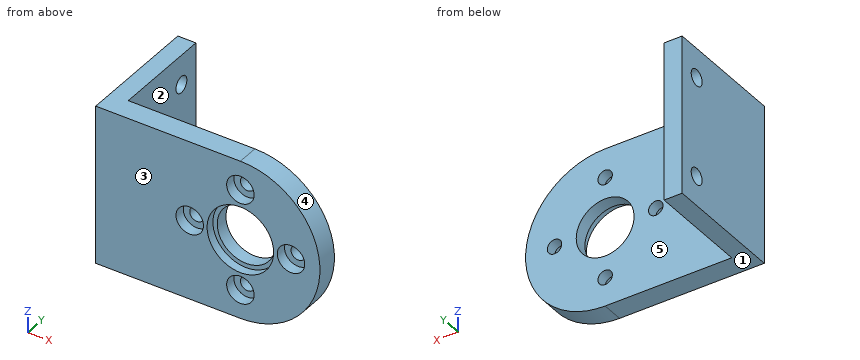
```python
from build123d import *

# Parameters (mm, degrees)
SKETCH1_R           = 1
SKETCH1_R_2         = 4
BOSS_EXTRUDE1_DEPTH = 3
SKETCH2_W           = 2.5
SKETCH2_H           = 22
BOSS_EXTRUDE2_DEPTH = 14
SKETCH3_R           = 1.132393425
SKETCH3_R_2         = 1.130977438
CUT_EXTRUDE1_DEPTH  = 6
SKETCH4_R           = 4.6
CUT_EXTRUDE2_DEPTH  = 1.2
SKETCH5_R           = 1.9
CUT_EXTRUDE3_DEPTH  = 1.5


with BuildPart() as part:
    # Sketch1 → Boss-Extrude1 (new body)
    with BuildSketch(Plane(origin=(0, 0, 0), x_dir=(1, 0, 0), z_dir=(0, 1, 0))):
        with BuildLine():
            Line((-14, -11), (-14, 11))
            Line((-14, 11), (6, 11))
            ThreePointArc((6, 11), (17, 0), (6, -11))
            Line((6, -11), (-14, -11))
        make_face()
        with Locations((6, -7)):
            Circle(SKETCH1_R, mode=Mode.SUBTRACT)
        with Locations((-1, 0)):
            Circle(SKETCH1_R, mode=Mode.SUBTRACT)
        with Locations((6, 0)):
            Circle(SKETCH1_R_2, mode=Mode.SUBTRACT)
        with Locations((13, 0)):
            Circle(SKETCH1_R, mode=Mode.SUBTRACT)
        with Locations((6, 7)):
            Circle(SKETCH1_R, mode=Mode.SUBTRACT)
    extrude(amount=BOSS_EXTRUDE1_DEPTH)

    # Sketch2 → Boss-Extrude2 (add)
    with BuildSketch(Plane(origin=(0, 3, 0), x_dir=(1, 0, 0), z_dir=(0, 1, 0))):
        with Locations((-12.75, 0)):
            Rectangle(SKETCH2_W, SKETCH2_H)
    extrude(amount=BOSS_EXTRUDE2_DEPTH)

    # Sketch3 → Cut-Extrude1 (cut)
    with BuildSketch(Plane(origin=(-11.5, 0, 0), x_dir=(0, 0, -1), z_dir=(1, 0, 0))):
        with Locations((6.9, 14)):
            Circle(SKETCH3_R)
        with Locations((-6.9, 14)):
            Circle(SKETCH3_R_2)
    extrude(amount=-CUT_EXTRUDE1_DEPTH, mode=Mode.SUBTRACT)

    # Sketch4 → Cut-Extrude2 (cut)
    with BuildSketch(Plane.XZ):
        with Locations((6, 0)):
            Circle(SKETCH4_R)
    extrude(amount=-CUT_EXTRUDE2_DEPTH, mode=Mode.SUBTRACT)

    # Sketch5 → Cut-Extrude3 (cut)
    with BuildSketch(Plane.XZ):
        with Locations((13, 0)):
            Circle(SKETCH5_R)
        with Locations((6, -7)):
            Circle(SKETCH5_R)
        with Locations((-1, 0)):
            Circle(SKETCH5_R)
        with Locations((6, 7)):
            Circle(SKETCH5_R)
    extrude(amount=-CUT_EXTRUDE3_DEPTH, mode=Mode.SUBTRACT)


solid = part.part
```
Source: CAD feature listing. Evaluate the final solid. Frame: model axes, mm. Face numbers are marked on the shaded views. A direction names the side the tool comes from. Coordinates: 2 decimals unless noted, no trailing zeros. Order: outer loops, then holes, each group sorted by start corner. A loop starts at its lowest first (then second) coordinate and runs counter-clockwise, first axis right, second up. Notation, with made-up numbers: (73, 40.5) - (132, 40.5) arc R6 cw to (132, 46.5) - close; hole circle Ø9 at (86, 14.5). An arc over 180 degrees is marked (long way). One line per item, written item: value.
1) Cut plane D-D on z = -2.25. Output: boundary loops of the cut face in (x, y), plus the area to 3 significant figures.
Computed values:
outline: (-14, 0) - (1.99, 0) - (1.99, 1.2) - (2.69, 1.2) - (2.69, 3) - (-11.5, 3) - (-11.5, 17) - (-14, 17) - close; (9.31, 1.2) - (10.01, 1.2) - (10.01, 0) - (16.77, 0) - (16.77, 3) - (9.31, 3) - close
area: 106 mm^2
2) Reachability of the marked faces 1 and 2 from +Z, -Z, +X, -X, +Y, -Y: full face, straight path, thin tool, end or side. Return the list, or none.
Computed values:
face 1: -Z, +X, -X, +Y, -Y
face 2: +Z, -Z, +X, +Y
3) Mould query, pull axis Y, two halves, no side actions, for the marked faces 3, 4 and 5. Classes: released by +Y, released by -Y, zero draft, split by the parting line, or undercut.
Computed values:
face 3: released by -Y
face 4: zero draft
face 5: released by +Y
4) Ray query, line 1 (Z direction, x = 6, y = 1.65); line 2 (X direction, y = 2.15, z = 0); line 3 (Y direction, x = -12.7, z = -6.9). Return the intervals inside material, ascending. Write a range as [from, to].
Computed values:
line 1: z = [-11, -8], [-6, -4], [4, 6], [8, 11]
line 2: x = [-14, -2], [0, 2], [10, 12], [14, 17]
line 3: y = [0, 12.87], [15.13, 17]
5) Cut plane C-C on x = 5.5. Output: boundary loops of the cut face in (y, z), plus the area to 3 significant figures.
Computed values:
outline: (0, -11) - (3, -11) - (3, -7.87) - (1.5, -7.87) - (1.5, -8.83) - (0, -8.83) - close; (0, -5.17) - (1.5, -5.17) - (1.5, -6.13) - (3, -6.13) - (3, -3.97) - (1.2, -3.97) - (1.2, -4.57) - (0, -4.57) - close; (0, 4.57) - (1.2, 4.57) - (1.2, 3.97) - (3, 3.97) - (3, 6.13) - (1.5, 6.13) - (1.5, 5.17) - (0, 5.17) - close; (0, 8.83) - (1.5, 8.83) - (1.5, 7.87) - (3, 7.87) - (3, 11) - (0, 11) - close
area: 24.5 mm^2
6) Contact query for flat-ended pins moving along their axis: pin 1 (3 mm diameter, centred on x = 13, z = 0, fed in from +Y); pin 2 (7 mm diameter, centred on x = 6, z = 0, fed in from -Y); pin 3 (3 mm diameter, centred on x = -1, z = 0, fed in from -Y); pin 4 (3 mm diameter, centred on y = 12.5, z = -2, fed in from +X). Output: stop coordinate, or through.
Computed values:
pin 1: stops at y = 3
pin 2: passes through
pin 3: stops at y = 1.5
pin 4: stops at x = -11.5
7) Cut plane B-B on y = 14. Output: boundary loops of the cut face in (x, z).
Computed values:
outline: (-14, -11) - (-11.5, -11) - (-11.5, -8.03) - (-14, -8.03) - close; (-14, -5.77) - (-11.5, -5.77) - (-11.5, 5.77) - (-14, 5.77) - close; (-14, 8.03) - (-11.5, 8.03) - (-11.5, 11) - (-14, 11) - close
8) Cut plane A-A on z = 7. Output: boundary loops of the cut face in (x, y), plus the area to 3 significant figures.
Computed values:
outline: (-14, 0) - (4.1, 0) - (4.1, 1.5) - (5, 1.5) - (5, 3) - (-11.5, 3) - (-11.5, 12.87) - (-14, 12.87) - close; (-14, 15.13) - (-11.5, 15.13) - (-11.5, 17) - (-14, 17) - close; (7, 1.5) - (7.9, 1.5) - (7.9, 0) - (14.49, 0) - (14.49, 3) - (7, 3) - close
area: 106 mm^2
